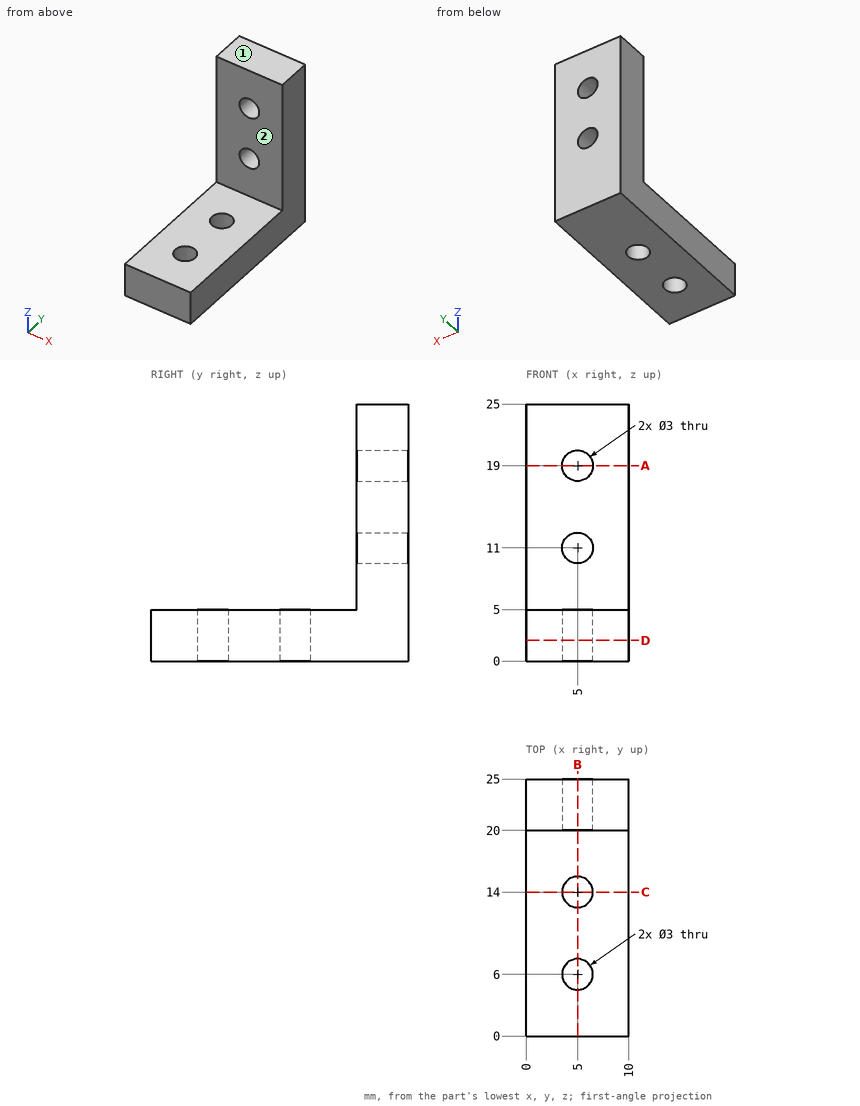
Can you work these out from the drawing? Everything is in mm from the part's minimum corner. A direction names the side the tool comes from. Give positions to 0.01 mm unless a question says otherwise; leave off trailing zeros. Loops run counter-clockwise (first coordinate to the right, second up) from the corner with the lowest first, then second, coordinate; pieces in that order, holes last. Notation, with made-up numbers: (-13.5, 43.5) -> (37.5, 43.5) arc R23 ccw to (37.5, 65.5) -> close; hole circle Ø11 at (-15.5, 80). An arc over 180 degrees is marked (long way). Write item = value, one per line.
1) Suppose I cut it at A-A on z = 19. Write out the boundary of the cut face in (x, y), then the cut area to 3 significant figures.
Check result:
outline = (0, 20) -> (3.5, 20) -> (3.5, 25) -> (0, 25) -> close; (6.5, 20) -> (10, 20) -> (10, 25) -> (6.5, 25) -> close
area = 35.0 mm2
2) I need wall thicknesses on L1, parallel to Y at x = 5, z = 1.45; L2, parallel to Z at x = 5, y = 23.4; L3, parallel to Y at x = 4.5, z = 13.25. Which ranges of each line are inside material? Lowest first, please. Write a range as from..to.
Check result:
L1 = 0..4.5, 7.5..12.5, 15.5..25
L2 = 0..9.5, 12.5..17.5, 20.5..25
L3 = 20..25
3) Suppose I cut it at C-C on y = 14. Write out the boundary of the cut face in (x, z).
Check result:
outline = (0, 0) -> (3.5, 0) -> (3.5, 5) -> (0, 5) -> close; (6.5, 0) -> (10, 0) -> (10, 5) -> (6.5, 5) -> close
4) Suppose I cut it at D-D on z = 2. Write out the boundary of the cut face in (x, y), then the cut area to 3 significant figures.
Check result:
outline = (0, 0) -> (10, 0) -> (10, 25) -> (0, 25) -> close; hole circle Ø3 at (5, 6); hole circle Ø3 at (5, 14)
area = 236 mm2
5) Will these pins go through, and if not, where does the flat tip stop? pin 1 (1.5 mm diameter, centred on x = 9, y = 5, fed in from +Z); pin 2 (4 mm diameter, centred on x = 5.5, z = 21.5, fed in from -Y).
Check result:
pin_1 = 5
pin_2 = 20
6) Suppose I cut it at B-B on x = 5. Write out the boundary of the cut face in (y, z), then the cut area to 3 significant figures.
Check result:
outline = (0, 0) -> (4.5, 0) -> (4.5, 5) -> (0, 5) -> close; (7.5, 0) -> (12.5, 0) -> (12.5, 5) -> (7.5, 5) -> close; (15.5, 0) -> (25, 0) -> (25, 9.5) -> (20, 9.5) -> (20, 5) -> (15.5, 5) -> close; (20, 12.5) -> (25, 12.5) -> (25, 17.5) -> (20, 17.5) -> close; (20, 20.5) -> (25, 20.5) -> (25, 25) -> (20, 25) -> close
area = 165 mm2
7) For the marked faces 1 and 2, which set-ups out of +Z, -Z, +X, -X, +Y, -Y let a thin tool reach every point of the face, with its end or its side?
Check result:
face_1 = +Z, +X, -X, +Y, -Y
face_2 = +Z, +X, -X, -Y
